Study the drawing (mm; zero at the part's minimum x, y, z) and answer. A direction names the side the tool comes from. Give positions to 0.01 mm unless a question says otherwise; leave off trailing zeros. Write each loop counter-clockwise with the first axis right and the second up, starting at its lowest first coordinate (ties: lowest second). Pieces come first, ordered by that corner, then holes. Notation, with made-up numbers: (-34.5, -16) - (-22.5, -16) arc R33 cw to (-22.5, 22) - close; hole circle Ø4 at (86, 6). An arc over 180 degrees is marked (long way). Answer in a Markdown table with one row per item. Add a question column.
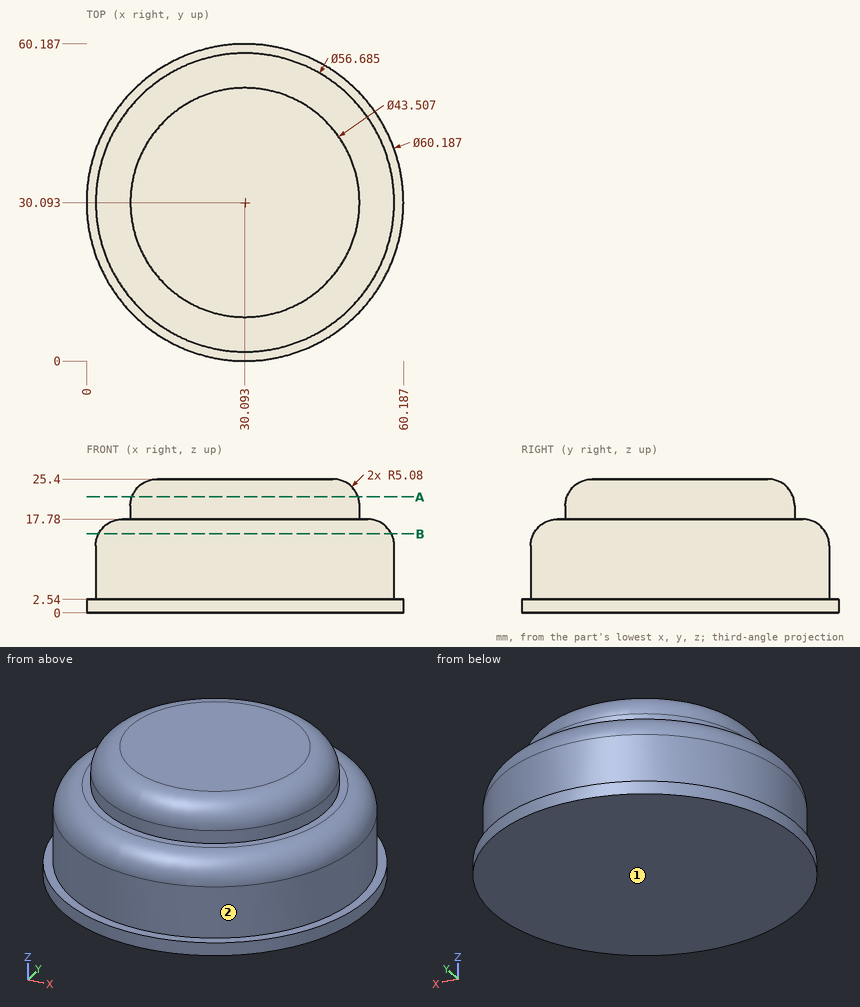
1. Section A-A (z = 22) is taken. Give the vertices of the cut face in (x, y) (1 decimal), and give its area (3 significant figures).
2. Straight lines are drawn through the part: L1, parallel to Y at x = 31, z = 3.5 (1 decimal); L2, parallel to Z at x = 46, y = 45.5; L3, parallel to Z at x = 10.5, y = 8. For each, find the intervals that lie inside material, in ascending order. Write a range as [from, to].
3. Section B-B (z = 15) is taken. Give the vertices of the cut face in (x, y) (1 decimal), and give its area (3 significant figures).
4. A tool of negligible diameter and unlimited length cuts with its end or side. For the marked faces 1 and 2, from which of +Z, -Z, +X, -X, +Y, -Y can it reach the whole face along a straight path? Write none if from no direction.
5. Given pin 1 Ø1 at (x, z) = (25, 3.5) entering from +Y; pin 2 Ø1 at (x, z) = (39, 12) entering from -Y; pin 3 Ø12 at (y, z) = (52.5, 12.5) entering from -X, each flat-ended and moving along its own axis, determine where each tip first touches the part or whether it passes through.
Geometry check:
| question | item | result |
|---|---|---|
| 1 | outline | circle Ø42.9 at (30.1, 30.1) |
| 1 | area | 1,450 mm² |
| 2 | L1 | [1.8, 58.4] |
| 2 | L2 | [0, 17.78] |
| 2 | L3 | [0, 2.54] |
| 3 | outline | circle Ø55.6 at (30.1, 30.1) |
| 3 | area | 2,430 mm² |
| 4 | face 1 | -Z, +X, -X, +Y, -Y |
| 4 | face 2 | +Z |
| 5 | pin 1 | y = 58.06 |
| 5 | pin 2 | y = 3.03 |
| 5 | pin 3 | x = 6.98 |
